```python
from build123d import *

# Parameters (mm, degrees)
CHANFREIN1_SIZE         = 0.5
ESQUISSE2_R             = 2.75
ENL_V_MAT_EXTRU_1_DEPTH = 90.297256397


with BuildPart() as part:
    # Esquisse1 → Révolution1 (revolve)
    with BuildSketch(Plane.XY, mode=Mode.PRIVATE) as r_volution1_sk:
        Polygon((0, 0), (25, 0), (25, 4), (15.632287961, 4), (7, 11.118702223), (5, 11.118702223), (5, 13.118702223), (3, 13.118702223), (3, 22), (4, 22), (4, 82), (0, 82), align=None)
    revolve(r_volution1_sk.sketch.rotate(Axis((0, 0, 0), (0, 1, 0)), 90), axis=Axis((0, 0, 0), (0, 1, 0)))

    # Chanfrein1
    chanfrein1_edges = [part.edges().sort_by_distance(p)[0] for p in [
        (0, 82, 4),
    ]]
    chamfer(chanfrein1_edges, length=CHANFREIN1_SIZE)

    # Esquisse2 → Enlèv. mat.-Extru.1 (cut, through all)
    with BuildSketch(Plane.XZ):
        with Locations(Location((-20, 0, 0), (0, 0, 270))):
            Circle(ESQUISSE2_R)
        with Locations(Location((20, 0, 0), (0, 0, 270))):
            Circle(ESQUISSE2_R)
    extrude(amount=-ENL_V_MAT_EXTRU_1_DEPTH, mode=Mode.SUBTRACT)


solid = part.part
```
Could you check a few things on this model? Use its own coordinates, in mm. A direction names the side the tool comes from. Round coordinates to 2 decimals unless told otherwise and drop trailing zeros. Write each loop counter-clockwise with the first axis right and the second up, starting at its lowest first coordinate (ties: lowest second). Pieces come first, ordered by that corner, then holes. Notation, with made-up numbers: M 16,75 L 70,75 A11 ccw 70,86 Z; hole C -14.5,23.5 d7. An arc over 180 degrees is marked long. Answer in a Markdown table with one row per item. Add a question column.
Q1. Imagine slicing it at D-D (y = 76). Please give me the cut outline in (x, z).
Q2. If I drill on line 1 (X direction, y = 1.4, z = 0); line 2 (Y direction, x = -14.5, z = -9.5); line 3 (Y direction, x = 1.5, z = -6), over which ranges is the centre line in solid material (lowest first)? Write a range as from..to.
Q3. Imagine slicing it at B-B (x = 0). Please give me the cut outline in (y, z).
Q4. Will these pins go through, and if not, where does the flat tip stop? pin 1 Ø2 at (x, z) = (-5.5, 9.5) entering from +Y; pin 2 Ø8 at (x, y) = (5, 43) entering from +Z; pin 3 Ø6 at (x, z) = (-11.5, 7.5) entering from +Y.
Q5. If we mould it in two halves opening along Y, with no side actions, what happens to faces 1 (the flat face through (-0.1, 13.119, -3.3)), 2 (the flat face through (-5, 11.119, 2)), 3 (the cylindrical face through (0, 12, 5))? For each: +Y half, -Y half, draft (parallel to the pull), parting line (faces both ways), or undercut.
Q6. Imagine slicing it at A-A (z = 0). Give the number of separate pieces and of enclosed holes in the cut face, then the cut area to 3 significant figures.
Q7. On a 3-axis mill with a long thin cutter (end or side, diameter ignored), from which of +Z, -Z, +X, -X, +Y, -Y can I reach the whole of each face in a straight line? I mean faces 4 (the cylindrical face through (3.905, 52.166, 0.867)), 5 (the flat face through (0, 0, 0)), 6 (the flat face through (-3, 22, 1)). Say none if no direction works.
Q8. Imagine slicing it at C-C (x = 20). Please give me the cut outline in (y, z).
Values:
| question | item | result |
|---|---|---|
| 1 | outline | C 0,0 d8 |
| 2 | line 1 | -25..-22.75, -17.25..17.25, 22.75..25 |
| 2 | line 2 | 0..4 |
| 2 | line 3 | 0..11.12 |
| 3 | outline | M 0,-25 L 4,-25 L 4,-15.63 L 11.12,-7 L 11.12,-5 L 13.12,-5 L 13.12,-3 L 22,-3 L 22,-4 L 81.5,-4 L 82,-3.5 L 82,3.5 L 81.5,4 L 22,4 L 22,3 L 13.12,3 L 13.12,5 L 11.12,5 L 11.12,7 L 4,15.63 L 4,25 L 0,25 Z |
| 4 | pin 1 | y = 8.66 |
| 4 | pin 2 | z = 3.87 |
| 4 | pin 3 | y = 8.04 |
| 5 | face 1 | undercut |
| 5 | face 2 | +Y half |
| 5 | face 3 | draft |
| 6 | separate pieces | 3 |
| 6 | enclosed holes | 0 |
| 6 | area | 870 mm^2 |
| 7 | face 4 | +Y |
| 7 | face 5 | +Z, -Z, +X, -X, -Y |
| 7 | face 6 | none |
| 8 | outline | M 0,-15 L 4,-15 L 4,-2.75 L 0,-2.75 Z; M 0,2.75 L 4,2.75 L 4,15 L 0,15 Z |
